Build history of the part. All positions in model axes, mm. A direction names the side the tool comes from. Round coordinates to 2 decimals unless told otherwise and drop trailing zeros. Use a Markdown table: item, result.
from build123d import *

# Parameters (mm, degrees)
SKETCH4_R          = 6.4643
SKETCH4_R_2        = 6.30555
CUT_EXTRUDE2_DEPTH = 4.064
CUT_EXTRUDE1_DEPTH = 4.064
CIRPATTERN1_COUNT  = 20
SKETCH6_R          = 1.5875
CUT_EXTRUDE3_DEPTH = 14.5020413
CIRPATTERN2_COUNT  = 2
CIRPATTERN2_ANGLE  = 90


with BuildPart() as part:
    # Sketch1 → Revolve1 (revolve)
    with BuildSketch(Plane.XY, mode=Mode.PRIVATE) as revolve1_sk:
        with BuildLine():
            Line((-5.5626, 3.175), (5.5626, 3.175))
            Line((5.5626, 3.175), (5.5626, 8.6995))
            Line((5.5626, 8.6995), (4.953, 8.6995))
            ThreePointArc((4.953, 8.6995), (4.500598199, 7.921733103), (4.3434, 7.0358))
            Line((4.3434, 7.0358), (4.3434, 6.4643))
            Line((4.3434, 6.4643), (0.2794, 6.4643))
            Line((0.2794, 6.4643), (0.2794, 7.6073))
            Line((0.2794, 7.6073), (-0.8128, 8.6995))
            Line((-0.8128, 8.6995), (-5.5626, 8.6995))
            Line((-5.5626, 8.6995), (-5.5626, 3.175))
        make_face()
    revolve(revolve1_sk.sketch.rotate(Axis((-5.5626, 0, 0), (1, 0, 0)), 90), axis=Axis((-5.5626, 0, 0), (1, 0, 0)))

    # Sketch4 → Cut-Extrude2 (cut)
    with BuildSketch(Plane(origin=(0.2794, 0, 0), x_dir=(0, 0, -1), z_dir=(1, 0, 0))):
        Circle(SKETCH4_R)
        Circle(SKETCH4_R_2, mode=Mode.SUBTRACT)
    extrude(amount=CUT_EXTRUDE2_DEPTH, mode=Mode.SUBTRACT)

    # Sketch3 → Cut-Extrude1 (cut)
    with BuildSketch(Plane(origin=(0.2794, 0, 0), x_dir=(0, 0, -1), z_dir=(1, 0, 0))):
        with BuildLine():
            Line((-0.642631898, 6.272717517), (-0.342185353, 5.628407823))
            Line((-0.342185353, 5.628407823), (0.342185353, 5.628407823))
            Line((0.342185353, 5.628407823), (0.642631898, 6.272717517))
            ThreePointArc((0.642631898, 6.272717517), (0, 6.30555), (-0.642631898, 6.272717517))
        make_face()
    cut_extrude1 = extrude(amount=CUT_EXTRUDE1_DEPTH, mode=Mode.SUBTRACT)

    # CirPattern1: Cut-Extrude1 ×20 about axis
    cirpattern1_axis = Axis((0, 0, 0), (1, 0, 0))
    for i in range(1, CIRPATTERN1_COUNT):
        add(cut_extrude1.rotate(cirpattern1_axis, i * 360 / CIRPATTERN1_COUNT), mode=Mode.SUBTRACT)

    # Sketch6 → Cut-Extrude3 (cut, through all)
    with BuildSketch(Plane(origin=(0, 0, 0), x_dir=(1, 0, 0), z_dir=(0, 1, 0))):
        with Locations(Location((-2.6416, 0, 0), (0, 0, 90))):
            Circle(SKETCH6_R)
    cut_extrude3 = extrude(amount=CUT_EXTRUDE3_DEPTH, mode=Mode.SUBTRACT)

    # CirPattern2: Cut-Extrude3 ×2 about axis
    cirpattern2_axis = Axis((-5.5626, 0, 0), (1, 0, 0))
    for i in range(1, CIRPATTERN2_COUNT):
        add(cut_extrude3.rotate(cirpattern2_axis, i * CIRPATTERN2_ANGLE / (CIRPATTERN2_COUNT - 1)), mode=Mode.SUBTRACT)


solid = part.part
Q1. Which spindle directions (+Z, -Z, +X, -X, +Y, -Y) get a long thin tool onto all of the face, cutting with end or side? Do faces 4 (the face through (-2.711, 5.685, 1.586)), 5 (the face through (-3.22, 8.49, -1.89)), 6 (the face through (-2.711, -1.586, 5.683)), 7 (the face through (5.563, 4, 0)), 8 (the face through (0.279, -2, 6)). Say none if no direction does.
Results found:
| item | result |
|---|---|
| face 4 | +Y |
| face 5 | +X, -X |
| face 6 | +Z |
| face 7 | +Z, -Z, +X, +Y, -Y |
| face 8 | none |
Q2. Pull direction X, two halves, no side cores. Call faces 1 (the face through (5.25, 8.49, -1.89)), 2 (the face through (-5.563, 4, 0)), 3 (the face through (4.343, -6, -2)): pulls with the +X half, pulls with the -X half, needs draft (parallel to the pull), parting line crosses it, or undercut.
Results found:
| item | result |
|---|---|
| face 1 | needs draft |
| face 2 | pulls with the -X half |
| face 3 | undercut |
Q3. Cut at A-A, the plane z = 0. Count the separate pieces of the cut face and the enclosed holes in it, plus the area to 3 significant figures.
Results found:
| item | result |
|---|---|
| separate pieces | 3 |
| enclosed holes | 0 |
| area | 78.6 mm2 |
Q4. Drop flat-ended pins along their axis: pin 1 (5.5 mm diameter, centred on y = 0, z = 0, fed in from -X); pin 2 (2 mm diameter, centred on x = 1, y = 6, fed in from +Z); pin 3 (1 mm diameter, centred on x = 3, z = 2, fed in from +Y); pin 4 (5 mm diameter, centred on x = -2.64, y = 0, fed in from +Z). Give the stop position or say it passes through.
Results found:
| item | result |
|---|---|
| pin 1 | passes through |
| pin 2 | stops at z = 5.47 |
| pin 3 | stops at y = 5.71 |
| pin 4 | stops at z = 8.7 |
Q5. Probe line 1 (X direction, y = 6.3, z = 0); line 2 (X direction, y = 4.5, z = 5.5); line 3 (Y direction, x = -2.75, z = 0.25). List the from-to ranges inside material, lowest first.
Results found:
| item | result |
|---|---|
| line 1 | x = -5.56 to -4.23, -1.05 to 0.28, 4.34 to 5.56 |
| line 2 | x = -5.56 to 0.28, 4.34 to 5.56 |
| line 3 | y = -8.7 to -3.17 |
